For this review, take the finished solid that the model builds, in its own axes (mm). Face numbers are marked on the shaded views. A direction names the side the tool comes from. Coordinates: 2 decimals unless noted, no trailing zeros. Loops run counter-clockwise (first coordinate to the right, second up) from the corner with the lowest first, then second, coordinate; pieces in that order, holes last. Notation, with made-up numbers: (-12.5, 12) - (38.5, 12) arc R11 ccw to (38.5, 28) - close; hole circle Ø3 at (37, 18.25). An arc over 180 degrees is marked (long way). Answer as a JSON object with one key per item and string values. Group by question number.
Item 1: We need section C-C (y = 12.5). Give the boundary of the cut face in (x, z).
Item 2: Mouldability with a two-part tool opening along X and no side actions: class the marked faces 4, 5 and 6 as released by +X, released by -X, zero draft, split by the parting line, or undercut.
Item 3: We need section B-B (x = 40). Give the boundary of the cut face in (y, z).
Item 4: We need section A-A (y = 3). State how many separate pieces and enclosed holes the cut face has, then the cut area to 3 significant figures.
Item 5: Tool access review of the marked faces 1, 2 and 3: name each direction out of +Z, -Z, +X, -X, +Y, -Y from which nothing blocks a thin tool from reaching the whole face with its end or side.
Item 6: To check wall thickness, follow line 1 (Y direction, x = 29, z = 11.5); line 2 (X direction, y = -8.5, z = 21); line 3 (X direction, y = -1, z = 30). State the ranges of each line that lie inside material, in increasing order.
Item 7: Clearance check with flat-ended pins moving along their axes: pin 1 (16 mm diameter, centred on y = 19.5, z = 41.5, fed in from -X); pin 2 (1 mm diameter, centred on x = 39, z = 11, fed in from -Y); pin 3 (12 mm diameter, centred on x = -37, z = 33.5, fed in from -Y). State where each tip first meets the part, or that it passes through.
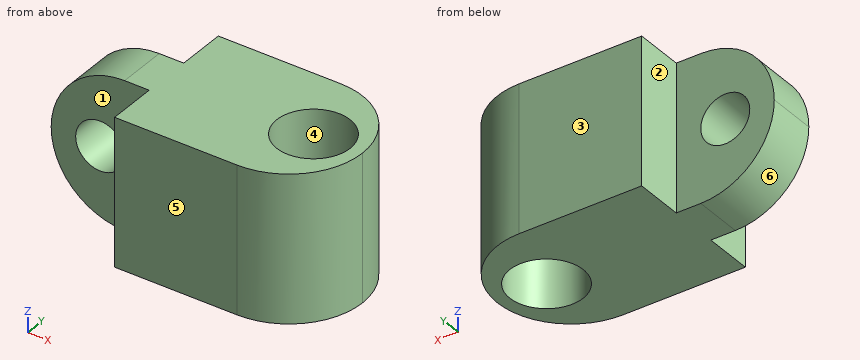
from build123d import *

# Parameters (mm, degrees)
CROQUIS4_W                 = 120
CROQUIS4_H                 = 60
SALIENTE_EXTRUIR3_DEPTH    = 60
REDONDEO1_R                = 30
CROQUIS5_W                 = 40
CROQUIS5_H                 = 20
CORTAR_EXTRUIR1_DEPTH      = 60
CORTAR_EXTRUIR2_DEPTH      = 10
CORTAR_EXTRUIR2_DEPTH_BACK = 10
CROQUIS6_R                 = 10
REDONDEO2_R                = 30
CROQUIS8_R                 = 15
CORTAR_EXTRUIR3_DEPTH      = 60


with BuildPart() as part:
    # Croquis4 → Saliente-Extruir3 (new body)
    with BuildSketch(Plane.XY):
        Rectangle(CROQUIS4_W, CROQUIS4_H)
    extrude(amount=SALIENTE_EXTRUIR3_DEPTH)

    # Redondeo1
    redondeo1_edges = [part.edges().sort_by_distance(p)[0] for p in [
        (60, -30, 30),
        (60, 30, 30),
    ]]
    fillet(redondeo1_edges, radius=REDONDEO1_R - 0.0001)  # a hair under: the kernel refuses the full size

    # Croquis5 → Cortar-Extruir1 (cut)
    with BuildSketch(Plane.XY):
        with Locations((-40, 20)):
            Rectangle(CROQUIS5_W, CROQUIS5_H)
        with Locations((-40, -20)):
            Rectangle(CROQUIS5_W, CROQUIS5_H)
    extrude(amount=CORTAR_EXTRUIR1_DEPTH, mode=Mode.SUBTRACT)

    # Croquis6 → Cortar-Extruir2 (cut, two sides: drawn at the far end of the back side and taken through both)
    with BuildSketch(Plane(origin=(0, 0, 0), x_dir=(1, 0, 0), z_dir=(0, 1, 0)).offset(-CORTAR_EXTRUIR2_DEPTH_BACK)):
        with Locations(Location((-40, -30, 0), (0, 0, 270))):
            Circle(CROQUIS6_R)
    extrude(amount=CORTAR_EXTRUIR2_DEPTH + CORTAR_EXTRUIR2_DEPTH_BACK, mode=Mode.SUBTRACT)

    # Redondeo2
    redondeo2_edges = [part.edges().sort_by_distance(p)[0] for p in [
        (-60, 0, 60),
        (-60, 0, 0),
    ]]
    fillet(redondeo2_edges, radius=REDONDEO2_R - 0.0001)  # a hair under: the kernel refuses the full size

    # Croquis8 → Cortar-Extruir3 (cut)
    with BuildSketch(Plane.XY):
        with Locations((40, 0)):
            Circle(CROQUIS8_R)
    extrude(amount=CORTAR_EXTRUIR3_DEPTH, mode=Mode.SUBTRACT)


solid = part.part
Check sheet entries:
{
 "1": {"outline": "(-20, 0) - (31.71, 0) - (31.71, 60) - (-20, 60) - close; (48.29, 0) - (57.27, 0) - (57.27, 60) - (48.29, 60) - close"},
 "2": {"face 4": "undercut", "face 5": "zero draft", "face 6": "released by -X"},
 "3": {"outline": "(-28.28, 0) - (-15, 0) - (-15, 60) - (-28.28, 60) - close; (15, 0) - (28.28, 0) - (28.28, 60) - (15, 60) - close"},
 "4": {"separate pieces": "2", "enclosed holes": "1", "area": "4,730 mm2"},
 "5": {"face 1": "+Z, -Z, -X, -Y", "face 2": "+Z, -Z, -X, +Y", "face 3": "+Z, -Z, +X, -X, +Y"},
 "6": {"line 1": "y = -30 to -10.2, 10.2 to 30", "line 2": "x = -58.62 to -44.36, -35.64 to 27.64, 52.36 to 58.77", "line 3": "x = -60 to -50, -30 to 25.03, 54.97 to 59.98"},
 "7": {"pin 1": "stops at x = -20", "pin 2": "stops at y = -28.77", "pin 3": "stops at y = -10"}
}
